For this review, take the finished solid that the model builds, in its own axes (mm). Face numbers are marked on the shaded views. A direction names the side the tool comes from. Give positions to 0.01 mm unless a question says otherwise; leave off trailing zeros. Write each loop counter-clockwise with the first axis right and the second up, starting at its lowest first coordinate (ties: lowest second). Pieces come first, ordered by that corner, then holes.
Q1. Mouldability with a two-part tool opening along Z and no side actions: class the marked faces 4, 5, 6 and 7 as released by +Z, released by -Z, zero draft, split by the parting line, or undercut.
Q2. We need section B-B (z = 0). Write out the cut boundary in (x, y), then the cut area to 3 significant figures.
Q3. For line 1 (Z direction, x = -0.5, y = 180); line 2 (X direction, y = 89.5, z = -27), list the stretches that pass through material, from the lowest coordinate up.
Q4. Machinability: for the marked faces 1, 2 and 3, which of the approach directions +Z, -Z, +X, -X, +Y, -Y give a long, thin tool a straight path to every point of the face, cutting with its end or side? Answer none if there is none.
Q5. We need section D-D (y = 0). Write out the cut boundary in (x, z), then the cut area to 3 significant figures.
Q6. We need section A-A (y = 180). Write out the cut boundary in (x, z), then the cut area to 3 significant figures.
Q7. Insertion check: P1, Ø4.5, axis at x = -22, z = -14, coming from the +Y side; P2, Ø18, axis at y = 76, z = -6, coming from the -X side; P3, Ø12, axis at x = -24.5, z = -13.5, coming from the -Y side. Each pin has a flat end and moves straight along its axis. Give the tip position at first contact, or say it passes through.
Q8. We need section C-C (x = 0). Write out the cut boundary in (y, z), then the cut area to 3 significant figures.
```python
from build123d import *

# Parameters (mm, degrees)
CROQUIS1_R              = 40
SALIENTE_EXTRUIR1_DEPTH = 30
CROQUIS2_W              = 60
CROQUIS2_H              = 100
SALIENTE_EXTRUIR2_DEPTH = 30
SALIENTE_EXTRUIR3_DEPTH = 15


with BuildPart() as part:
    # Croquis1 → Saliente-Extruir1 (new, symmetric)
    with BuildSketch(Plane.XY):
        Circle(CROQUIS1_R)
    extrude(amount=SALIENTE_EXTRUIR1_DEPTH, both=True)

    # Croquis2 → Saliente-Extruir2 (add, symmetric)
    with BuildSketch(Plane.XY):
        with Locations((0, 50)):
            Rectangle(CROQUIS2_W, CROQUIS2_H)
    extrude(amount=SALIENTE_EXTRUIR2_DEPTH, both=True)

    # Croquis3 → Saliente-Extruir3 (add, symmetric)
    with BuildSketch(Plane(origin=(0, 0, 0), x_dir=(0, 0, -1), z_dir=(1, 0, 0))):
        with BuildLine():
            Line((-30, 130), (-30, 100))
            Line((-30, 100), (30, 100))
            Line((30, 100), (30, 130))
            Line((30, 130), (50, 160))
            Line((50, 160), (50, 200))
            Line((50, 200), (30, 280))
            Line((30, 280), (10, 280))
            Line((10, 280), (10, 202.912878475))
            ThreePointArc((10, 202.912878475), (0, 155), (-10, 202.912878475))
            Line((-10, 202.912878475), (-10, 280))
            Line((-10, 280), (-30, 280))
            Line((-30, 280), (-50, 200))
            Line((-50, 200), (-50, 160))
            Line((-50, 160), (-30, 130))
        make_face()
    extrude(amount=SALIENTE_EXTRUIR3_DEPTH, both=True)


solid = part.part
```
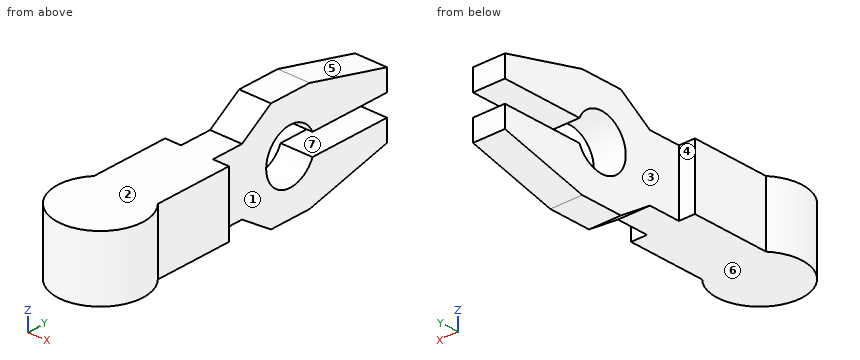
Computed:
1. face 4: zero draft
1. face 5: released by +Z
1. face 6: released by -Z
1. face 7: undercut
2. outline: (-30, 26.46) arc R40 ccw (long way) to (30, 26.46) - (30, 100) - (15, 100) - (15, 155) - (-15, 155) - (-15, 100) - (-30, 100) - close
2. area: 10,500 mm2
3. line 1: z = -50 to -25, 25 to 50
3. line 2: x = -30 to 30
4. face 1: +Z, -Z, +X, +Y
4. face 2: +Z, +X, -X, -Y
4. face 3: +Z, -Z, -X, +Y
5. outline: (-40, -30) - (40, -30) - (40, 30) - (-40, 30) - close
5. area: 4,800 mm2
6. outline: (-15, -50) - (15, -50) - (15, -25) - (-15, -25) - close; (-15, 25) - (15, 25) - (15, 50) - (-15, 50) - close
6. area: 1,500 mm2
7. P1: stops at y = 100
7. P2: stops at x = -30
7. P3: stops at y = -35.46
8. outline: (-40, -30) - (130, -30) - (160, -50) - (200, -50) - (280, -30) - (280, -10) - (202.91, -10) arc R25 cw (long way) to (202.91, 10) - (280, 10) - (280, 30) - (200, 50) - (160, 50) - (130, 30) - (-40, 30) - close
8. area: 19,500 mm2
